Can you work these out from the model? Positions are in its coordinate system, mm. Face numbers are marked on the shaded views. A direction names the side the tool comes from. Coordinates: 2 decimals unless noted, no trailing zeros. Write each loop counter-clockwise with the first axis right and the second up, starting at its lowest first coordinate (ties: lowest second). Pieces come first, ordered by that corner, then holes. Notation, with made-up numbers: (27.25, -15.5) - (35.25, -15.5) arc R20 cw to (35.25, 10.5) - close; hole circle Ø6 at (-1, 31.5). An arc over 180 degrees is marked (long way). Write each question's results on one line, items separated by ' | '. Start each with the question number.
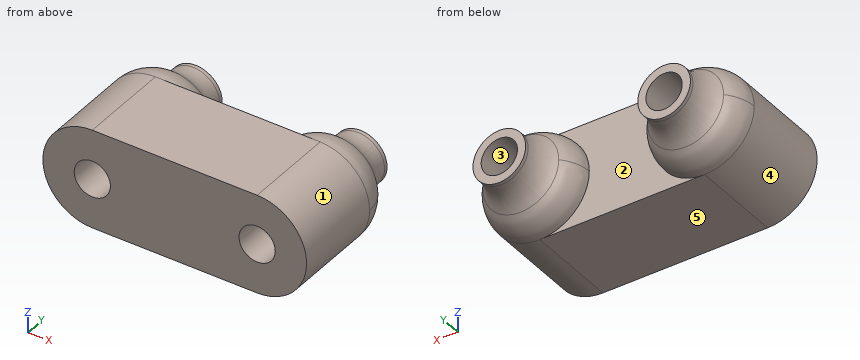
Autodesk Inventor part; units mm, degrees
ref_plane "XZ Plane" through (0, 0, 0) normal (0, 1, 0) x (-1, 0, 0)
ref_plane "XY Plane" through (0, 0, 0) normal (0, 0, 1) x (1, 0, 0)
sketch "Sketch1" plane through (0, 0, 0) normal (0, 1, 0) x (-1, 0, 0)
  circle A0 centre (0, 0) radius 7.5
  circle A1 centre (0, 0) radius 2.75
  dimension "d0" = 15
  dimension "d1" = 5.5
extrude "Extrusion1" add sketch "Sketch1" along normal blind 17
sketch "Sketch2" plane through (0, 17, 0) normal (0, 1, 0) x (1, 0, 0)
  circle A0 centre (0, 0) radius 2.75
  circle A1 centre (0, 0) radius 2.75
  circle A2 centre (0, 0) radius 4
  dimension "d4" = 5.5
  dimension "d5" = 8
extrude "Extrusion2" add sketch "Sketch2" along normal blind 6
fillet "Fillet1" radius 6 1 edges at (-4, 17, 0)
fillet "Fillet2" radius 6 2 edges at (0, 17, -7.5) (0, 17, 7.5)
ref_plane "Work Plane1" through (12.5, 0, 0) normal (1, 0, 0) x (0, 1, 0)
mirror "Mirror1" about plane through (12.5, 0, 0) normal (1, 0, 0) of "Extrusion1", "Extrusion2", "Fillet1", "Fillet2"
sketch "Sketch3" plane through (0, 0, 0) normal (0, 1, 0) x (-1, 0, 0)
  circle A0 centre (-25, 0) radius 2.75
  line L0 (-25, 0) -> (-25, 2.75)
  line L1 (-25, 0) -> (-25, -2.75)
  line L2 (0, 0) -> (0, -2.75)
  circle A1 centre (0, 0) radius 2.75
  line L3 (0, 0) -> (0, 2.75)
  line L4 (-25, 2.75) -> (0, 2.75)
  line L5 (0, 2.75) -> (0, 7.5)
  line L6 (0, 7.5) -> (-25, 7.5)
  line L7 (-25, 7.5) -> (-25, 2.75)
  line L8 (-25, -2.75) -> (0, -2.75)
  line L9 (0, -2.75) -> (0, -7.5)
  line L10 (0, -7.5) -> (-25, -7.5)
  line L11 (-25, -7.5) -> (-25, -2.75)
  dimension "d11" = 25
  dimension "d12" = 4.75
  dimension "d13" = 25
  dimension "d14" = 4.75
extrude "Extrusion3" add sketch "Sketch3" along normal blind 14 contours A0 L4 A1 L8 | L7 L6 L5 L4 | L8 L9 L10 L11
properties part number "4mm_Roller_Spacer_simple3mm"
Q1. Thinking about a two-plate mould opening in X: for the marked faces 3, 4 and 5, which applies, pulls with the +X half, pulls with the -X half, needs draft (parallel to the pull), parting line crosses it, or undercut?
Q2. I need wall thicknesses on line 1 along X through (y, z) = (7.75, 0); line 2 along Z through (x, y) = (25, 11.75); line 3 along Y through (x, z) = (7, 6.25). Which ranges of each line are inside material? Lowest first, please. Write a range as from..to.
Q3. If we section it at B-B (x = 14.5): Please give me the cut outline in (y, z).
Q4. I'm going to push flat-ended pins straight in: pin 1 Ø4 at (x, z) = (20, 4.5) entering from +Y; pin 2 Ø4 at (y, z) = (2.5, 3.5) entering from -X; pin 3 Ø2 at (y, z) = (14.5, 1.5) entering from +X. Where does each tip first touch, or does it pass through?
Q5. If we section it at A-A (y = 1.5): Please give me the cut outline in (x, z).
Q6. For the marked faces 1 and 2, which set-ups out of +Z, -Z, +X, -X, +Y, -Y let a thin tool reach every point of the face, with its end or its side?
Answer list:
1) face 3: undercut | face 4: pulls with the -X half | face 5: needs draft
2) line 1: x = -7.5..-2.75, 2.75..22.25, 27.75..32.5 | line 2: z = -7.5..-2.75, 2.75..7.5 | line 3: y = 0..14
3) outline: (0, -7.5) - (14, -7.5) - (14, 7.5) - (0, 7.5) - close
4) pin 1: stops at y = 19.59 | pin 2: stops at x = -7.35 | pin 3: stops at x = 32.48
5) outline: (0, -7.5) - (25, -7.5) arc R7.5 ccw to (25, 7.5) - (0, 7.5) arc R7.5 ccw to start; hole circle Ø5.5 at (0, 0); hole circle Ø5.5 at (25, 0)
6) face 1: +X, +Y, -Y | face 2: +Y
